Source: CAD feature listing. Evaluate the final solid. Frame: model axes, mm. A direction names the side the tool comes from. Coordinates: 2 decimals unless noted, no trailing zeros. Write each loop counter-clockwise with the first axis right and the second up, starting at its lowest first coordinate (ties: lowest second). Pieces come first, ordered by that corner, then holes. Notation, with made-up numbers: (27, -37) - (41, -37) arc R17 ccw to (41, -6) - close; hole circle Ø5 at (55, 2.25). An arc over 180 degrees is marked (long way). One line per question, with ' | ' between items. Start each with the question number.
Q1. Cut plane B-B, the plane x = -23.75. Return loops of the section in (y, z), plus the area to 3 significant figures.
Q2. Draft query along Y for faces 4 (the face through (-50, -8, 8)), 5 (the face through (-38.82, -49.93, 6.94)), 6 (the face through (-38, -45, 5)). Return one class per face: +Y half, -Y half, draft (parallel to the pull), parting line (faces both ways), or undercut.
Q3. Cut plane A-A, the plane y = -50. Return loops of the section in (x, z).
Q4. Cut plane C-C, the plane z = 2. Return loops of the section in (x, y), plus the area to 3 significant figures.
Q5. Contact query for flat-ended pins moving along their axis: P1, Ø3, axis at x = -69.5, y = -3.5, coming from the -Z side; P2, Ø2, axis at y = -19.5, z = 10.5, coming from the +X side; P3, Ø3.5, axis at x = -23.75, z = 7, coming from the +Y side. Output: stop coordinate, or through.
Q6. Line query: line 1 (Y direction, x = -70, z = 12.85); line 2 (Y direction, x = -27, z = 11.5); line 3 (Z direction, x = -37.5, y = -9). Output: solid intervals per line, ascending.
Q7. Access query for faces 1 (the face through (-66.753, -4.857, 5.916)), 2 (the face through (-48.15, -3.94, 6.02)), 3 (the face through (-3.4, -6.2, 13)). Directions: +Z, -Z, +X, -X, +Y, -Y. A direction counts if a zero-diameter tool reaches every point of the face in a straight line with its end or side. Return the directions, or none.
Q8. Cut plane D-D, the plane z = 7. Give the number of separate pieces and of enclosed holes in the cut face, plus the area to 3 significant figures.
```python
from build123d import *

# Parameters (mm, degrees)
SKETCH2_W               = 75
SKETCH2_H               = 55
SKETCH2_W_2             = 55
SKETCH2_H_2             = 35
BOSS_EXTRUDE1_DEPTH     = 12
SKETCH3_W               = 75
SKETCH3_H               = 55
BOSS_EXTRUDE2_DEPTH     = 2
SKETCH5_R               = 1.32
CUT_EXTRUDE1_DEPTH      = 46
CUT_EXTRUDE1_DEPTH_BACK = 11
SKETCH6_R               = 3.25
CUT_EXTRUDE2_DEPTH      = 8
SKETCH8_R               = 3.25
CUT_EXTRUDE4_DEPTH      = 12
SKETCH9_R               = 2
CUT_EXTRUDE5_DEPTH      = 15


with BuildPart() as part:
    # Sketch2 → Boss-Extrude1 (new body)
    with BuildSketch(Plane.XY):
        with Locations((-37.5, -27.5)):
            Rectangle(SKETCH2_W, SKETCH2_H)
        with Locations((-37.5, -27.5)):
            Rectangle(SKETCH2_W_2, SKETCH2_H_2, mode=Mode.SUBTRACT)
    extrude(amount=BOSS_EXTRUDE1_DEPTH)

    # Sketch3 → Boss-Extrude2 (add)
    with BuildSketch(Plane.XY.offset(12)):
        with Locations((-37.5, -27.5)):
            Rectangle(SKETCH3_W, SKETCH3_H)
    extrude(amount=BOSS_EXTRUDE2_DEPTH)

    # Sketch5 → Cut-Extrude1 (cut, two sides)
    with BuildSketch(Plane(origin=(0, -45, 0), x_dir=(1, 0, 0), z_dir=(0, 1, 0))) as cut_extrude1_sk:
        with Locations((-51.25, -7)):
            Circle(SKETCH5_R)
        with Locations((-23.75, -7)):
            Circle(SKETCH5_R)
        with Locations((-37.5, -7)):
            Circle(SKETCH5_R)
    extrude(amount=CUT_EXTRUDE1_DEPTH, mode=Mode.SUBTRACT)
    extrude(cut_extrude1_sk.sketch, amount=-CUT_EXTRUDE1_DEPTH_BACK, mode=Mode.SUBTRACT)

    # Sketch6 → Cut-Extrude2 (cut)
    with BuildSketch(Plane(origin=(0, 0, 0), x_dir=(1, 0, 0), z_dir=(0, 1, 0))):
        with Locations((-51.25, -7)):
            Circle(SKETCH6_R)
        with Locations((-37.5, -7)):
            Circle(SKETCH6_R)
        with Locations((-23.75, -7)):
            Circle(SKETCH6_R)
    extrude(amount=-CUT_EXTRUDE2_DEPTH, mode=Mode.SUBTRACT)

    # Sketch8 → Cut-Extrude4 (cut)
    with BuildSketch(Plane(origin=(0, 0, 0), x_dir=(-1, 0, 0), z_dir=(0, 0, -1))):
        with Locations((5, -5)):
            Circle(SKETCH8_R)
        with Locations((70, -5)):
            Circle(SKETCH8_R)
        with Locations((70, -50)):
            Circle(SKETCH8_R)
        with Locations((5, -50)):
            Circle(SKETCH8_R)
    extrude(amount=-CUT_EXTRUDE4_DEPTH, mode=Mode.SUBTRACT)

    # Sketch9 → Cut-Extrude5 (cut, through all)
    with BuildSketch(Plane(origin=(0, 0, 0), x_dir=(-1, 0, 0), z_dir=(0, 0, -1))):
        with Locations((5, -5)):
            Circle(SKETCH9_R)
        with Locations((70, -5)):
            Circle(SKETCH9_R)
        with Locations((70, -50)):
            Circle(SKETCH9_R)
        with Locations((5, -50)):
            Circle(SKETCH9_R)
    extrude(amount=-CUT_EXTRUDE5_DEPTH, mode=Mode.SUBTRACT)


solid = part.part
```
Reply:
1) outline: (-55, 0) - (-45, 0) - (-45, 5.68) - (-55, 5.68) - close; (-55, 8.32) - (-45, 8.32) - (-45, 12) - (-10, 12) - (-10, 8.32) - (-8, 8.32) - (-8, 10.25) - (0, 10.25) - (0, 14) - (-55, 14) - close; (-10, 0) - (0, 0) - (0, 3.75) - (-8, 3.75) - (-8, 5.68) - (-10, 5.68) - close | area: 266 mm^2
2) face 4: +Y half | face 5: draft | face 6: undercut
3) outline: (-75, 0) - (-73.25, 0) - (-73.25, 12) - (-72, 12) - (-72, 14) - (-75, 14) - close; (-68, 12) - (-66.75, 12) - (-66.75, 0) - (-8.25, 0) - (-8.25, 12) - (-7, 12) - (-7, 14) - (-68, 14) - close; (-3, 12) - (-1.75, 12) - (-1.75, 0) - (0, 0) - (0, 14) - (-3, 14) - close; hole circle Ø2.64 at (-51.25, 7); hole circle Ø2.64 at (-37.5, 7); hole circle Ø2.64 at (-23.75, 7)
4) outline: (-75, -55) - (0, -55) - (0, 0) - (-75, 0) - close; hole circle Ø6.5 at (-70, -50); hole circle Ø6.5 at (-70, -5); hole (-65, -45) - (-10, -45) - (-10, -10) - (-65, -10) - close; hole circle Ø6.5 at (-5, -50); hole circle Ø6.5 at (-5, -5) | area: 2,070 mm^2
5) P1: stops at z = 12 | P2: stops at x = 0 | P3: stops at y = -8
6) line 1: y = -55 to -52, -48 to -7, -3 to 0 | line 2: y = -55 to -45, -10 to 0 | line 3: z = 0 to 5.68, 8.32 to 14
7) face 1: -Z | face 2: +Y | face 3: +Z, -Z
8) separate pieces: 6 | enclosed holes: 4 | area: 1,820 mm^2
